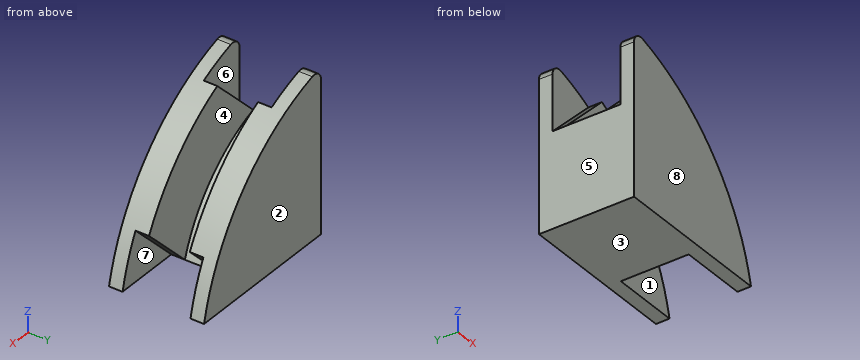
```python
from build123d import *

# Parameters (mm, degrees)
F1_DEPTH = 3.5
F3_DEPTH = 1.5
F5_DEPTH = 2.5
F6_R     = 0.7


with BuildPart() as f1:
    # F0 (on Front) → F1 (new body, symmetric)
    with BuildSketch(Plane.XZ):
        with BuildLine():
            ThreePointArc((15.5, 3.5), (11.2361025271, 11.2361025271), (3.5, 15.5))
            Line((3.5, 15.5), (3.5, 3.5))
            Line((3.5, 3.5), (15.5, 3.5))
        make_face()
    extrude(amount=F1_DEPTH, both=True)

    # F2 (on Front) → F3 (cut, symmetric)
    with BuildSketch(Plane.XZ):
        with BuildLine():
            ThreePointArc((3.5, 10.5), (7.8262379212, 7.8262379212), (10.5, 3.5))
            Line((10.5, 3.5), (15.5, 3.5))
            ThreePointArc((15.5, 3.5), (11.2361025271, 11.2361025271), (3.5, 15.5))
            Line((3.5, 15.5), (3.5, 10.5))
        make_face()
    extrude(amount=F3_DEPTH, both=True, mode=Mode.SUBTRACT)

    # F4 (on Front) → F5 (cut, symmetric)
    with BuildSketch(Plane.XZ):
        with BuildLine():
            ThreePointArc((7.177078252, 14.177078252), (5.3793615316, 14.9520055348), (3.5, 15.5))
            Line((3.5, 15.5), (3.5, 10.5))
            Line((3.5, 10.5), (7.177078252, 14.177078252))
        make_face()
        with BuildLine():
            Line((14.177078252, 7.177078252), (10.5, 3.5))
            Line((10.5, 3.5), (15.5, 3.5))
            ThreePointArc((15.5, 3.5), (14.9520055348, 5.3793615316), (14.177078252, 7.177078252))
        make_face()
    extrude(amount=F5_DEPTH, both=True, mode=Mode.SUBTRACT)

    # F6
    f6_edges = [f1.edges().sort_by_distance(p)[0] for p in [
        (3.5, 3, 15.5),
        (3.5, -3, 15.5),
    ]]
    fillet(f6_edges, radius=F6_R)


solid = f1.part
```
Source: CAD feature listing. Evaluate the final solid. Frame: model axes, mm. Face numbers are marked on the shaded views. A direction names the side the tool comes from. Give positions to 0.01 mm unless a question says otherwise; leave off trailing zeros. Write each loop counter-clockwise with the first axis right and the second up, starting at its lowest first coordinate (ties: lowest second). Pieces come first, ordered by that corner, then holes.
1. Section query C-C (y = 2). Return the cut outline in (x, z).
2. Section query D-D (z = 8.75). Return the cut outline in (x, y), then the cut area to 3 significant figures.
3. Pull-direction query (Y, two-part tool) for the marked faces 1, 2 and 3; classes: +Y half, -Y half, draft (parallel to the pull), parting line (faces both ways), or undercut.
4. Access query for the marked faces 4, 5, 6, 7 and 8. Directions: +Z, -Z, +X, -X, +Y, -Y. A direction counts if a zero-diameter tool reaches every point of the face in a straight line with its end or side. Return the directions, or none.
5. First-contact query: pin 1 (3 mm diameter, centred on x = 10.5, y = 2.5, fed in from +Z); pin 2 (2 mm diameter, centred on x = 10.5, y = 1, fed in from +Z). Flat tips, straight axial feed; report the tip coordinate or a pass-through.
6. Section query B-B (z = 11). Return the cut outline in (x, y), then the cut area to 3 significant figures.
7. Section query A-A (x = 11). Return the cut outline in (y, z).
8. Material intervals for line 1 along Y through (x, z) = (13.25, 4.5); line 2 along Y through (x, z) = (5.5, 11.25); line 3 along Z through (x, y) = (7, -1.25), sorted ascending.
Output values:
1. outline: (3.5, 3.5) - (10.5, 3.5) - (14.18, 7.18) arc R15.89 ccw to (7.18, 14.18) - (3.5, 10.5) - close
2. outline: (3.5, -3.5) - (13.26, -3.5) - (13.26, -1.5) - (6.78, -1.5) - (6.78, 1.5) - (13.26, 1.5) - (13.26, 3.5) - (3.5, 3.5) - close
2. area: 48.9 mm2
3. face 1: undercut
3. face 2: +Y half
3. face 3: draft
4. face 4: +Z, +X
4. face 5: +Z, -Z, -X, +Y, -Y
4. face 6: +Z, -X
4. face 7: -Z, +X
4. face 8: +Z, -Z, +X, -X, -Y
5. pin 1: stops at z = 13.1
5. pin 2: stops at z = 12.64
6. outline: (3.5, -3.5) - (11.47, -3.5) - (11.47, -1.5) - (4, -1.5) - (4, -2.5) - (3.5, -2.5) - close; (3.5, 2.5) - (4, 2.5) - (4, 1.5) - (11.47, 1.5) - (11.47, 3.5) - (3.5, 3.5) - close
6. area: 30.9 mm2
7. outline: (-3.5, 3.5) - (-2.5, 3.5) - (-2.5, 4) - (-1.5, 4) - (-1.5, 11.47) - (-3.5, 11.47) - close; (1.5, 4) - (2.5, 4) - (2.5, 3.5) - (3.5, 3.5) - (3.5, 11.47) - (1.5, 11.47) - close
8. line 1: y = -3.5 to -2.5, 2.5 to 3.5
8. line 2: y = -3.5 to -1.5, 1.5 to 3.5
8. line 3: z = 3.5 to 8.57
